Autodesk Inventor part; units mm, degrees
ref_plane "Work Plane1" through (0, 13.97, 1.5) normal (0, 1, 0) x (1, 0, 0)
ref_plane "YZ Plane" through (0, 0, 0) normal (1, 0, 0) x (0, 1, 0)
ref_plane "XZ Plane" through (0, 0, 0) normal (0, 1, 0) x (-1, 0, 0)
sketch "Sketch1" plane through (0, 0, 0) normal (0, 0, 1) x (1, 0, 0)
  line L0 (0, 0) -> (18.04, 0)
  line L1 (18.04, 0) -> (18.04, 27.94) construction
  line L2 (18.04, 27.94) -> (0, 27.94)
  line L3 (0, 27.94) -> (0, 0) construction
  circle A0 centre (9.02, 26.94) radius 0.32
  circle A1 centre (6.48, 26.94) radius 0.32
  circle A2 centre (3.94, 26.94) radius 0.32
  circle A3 centre (11.56, 26.94) radius 0.32
  circle A4 centre (14.1, 26.94) radius 0.32
  circle A5 centre (9.02, 1) radius 0.32
  circle A6 centre (6.48, 1) radius 0.32
  circle A7 centre (3.94, 1) radius 0.32
  circle A8 centre (11.56, 1) radius 0.32
  circle A9 centre (14.1, 1) radius 0.32
  line L4 (-2.665, 23.07) -> (20.705, 23.07) construction
  line L5 (20.705, 23.07) -> (20.705, 4.87) construction
  line L6 (20.705, 4.87) -> (-2.665, 4.87) construction
  line L7 (-2.665, 4.87) -> (-2.665, 23.07) construction
  line L8 (0, 27.94) -> (0, 23.07)
  line L9 (0, 23.07) -> (-2.665, 23.07)
  line L10 (-2.665, 23.07) -> (-2.665, 4.87)
  line L11 (-2.665, 4.87) -> (0, 4.87)
  line L12 (0, 0) -> (0, 4.87)
  line L13 (18.04, 0) -> (18.04, 4.87)
  line L14 (18.04, 4.87) -> (20.705, 4.87)
  line L15 (20.705, 4.87) -> (20.705, 23.07)
  line L16 (20.705, 23.07) -> (18.04, 23.07)
  line L17 (18.04, 23.07) -> (18.04, 27.94)
  point P0 (9.02, 27.94)
  point P1 (9.02, 23.07)
  point P2 (18.04, 13.97)
  point P3 (20.705, 13.97)
  dimension "d0" = 18.04
  dimension "d1" = 27.94
  dimension "d2" = 0.64
  dimension "d3" = 0.64
  dimension "d4" = 2.54
  dimension "d5" = 0.64
  dimension "d6" = 0.64
  dimension "d7" = 0.64
  dimension "d8" = 2.54
  dimension "d9" = 2.54
  dimension "d10" = 2.54
  dimension "d11" = 1
  dimension "d12" = 0.64
  dimension "d13" = 0.64
  dimension "d14" = 2.54
  dimension "d15" = 0.64
  dimension "d16" = 0.64
  dimension "d17" = 0.64
  dimension "d18" = 2.54
  dimension "d19" = 2.54
  dimension "d20" = 2.54
  dimension "d21" = 1
  dimension "d24" = 23.37
  dimension "d25" = 18.2
extrude "Extrusion1" add sketch "Sketch1" along normal blind 1.5
sketch "Sketch2" plane through (0, 0, 1.5) normal (0, 0, 1) x (1, 0, 0)
  line L0 (-2.565, 25.07) -> (20.605, 25.07)
  line L1 (20.605, 25.07) -> (20.605, 2.87)
  line L2 (20.605, 2.87) -> (-2.565, 2.87)
  line L3 (-2.565, 2.87) -> (-2.565, 25.07)
  line L4 (-2.665, 23.07) -> (-2.665, 4.87)
  line L5 (20.705, 4.87) -> (20.705, 23.07)
  line L6 (18.04, 27.94) -> (0, 27.94)
  point P0 (0, 0)
  point P1 (9.02, 25.07)
  point P2 (9.02, 27.94)
  dimension "d27" = 22.2
  dimension "d30" = 0.1
extrude "Extrusion2" add sketch "Sketch2" along normal blind 5.51
sketch "Sketch3" plane through (0, 0, 1.5) normal (0, 0, -1) x (-1, 0, 0)
  line L0 (0, 23.07) -> (2.565, 23.07)
  line L1 (2.565, 23.07) -> (2.565, 25.07)
  line L2 (2.565, 25.07) -> (0, 25.07)
  line L3 (0, 25.07) -> (0, 23.07)
  line L4 (0, 4.87) -> (0, 2.87)
  line L5 (0, 2.87) -> (2.565, 2.87)
  line L6 (2.565, 2.87) -> (2.565, 4.87)
  line L7 (2.565, 4.87) -> (0, 4.87)
  line L8 (-20.605, 23.07) -> (-18.04, 23.07)
  line L9 (-18.04, 23.07) -> (-18.04, 25.07)
  line L10 (-18.04, 25.07) -> (-20.605, 25.07)
  line L11 (-20.605, 25.07) -> (-20.605, 23.07)
  line L12 (-18.04, 2.87) -> (-18.04, 4.87)
  line L13 (-18.04, 4.87) -> (-20.605, 4.87)
  line L14 (-20.605, 4.87) -> (-20.605, 2.87)
  line L15 (-20.605, 2.87) -> (-18.04, 2.87)
  point P0 (0, 0)
extrude "Extrusion3" add sketch "Sketch3" along normal blind 3
sketch "Sketch4" plane through (0, 0, 7.01) normal (0, 0, 1) x (1, 0, 0)
  circle A0 centre (9.02, 13.97) radius 4.5
  line L0 (20.605, 25.07) -> (-2.565, 25.07) construction
  line L1 (-2.565, 25.07) -> (-2.565, 2.87) construction
  line L2 (-2.565, 2.87) -> (20.605, 2.87) construction
  line L3 (20.605, 2.87) -> (20.605, 25.07) construction
  point P0 (0, 0)
  point P1 (9.02, 25.07)
  point P2 (20.605, 13.97)
  dimension "d33" = 9
extrude "Extrusion4" add sketch "Sketch4" along normal blind 6.35
sketch "Sketch5" plane through (9.02, 13.97, 13.36) normal (0, 0, 1) x (1, 0, 0)
  circle A0 centre (0, 0) radius 3.16
  circle A1 centre (0, 0) radius 4.5 construction
  point P0 (-9.02, -13.97)
  dimension "d36" = 6.32
extrude "Extrusion5" add sketch "Sketch5" along normal blind 12.7
sketch "Sketch6" plane through (9.02, 13.97, 26.06) normal (0, 0, 1) x (1, 0, 0)
  line L0 (-3.16, 0.595) -> (3.16, 0.595)
  line L1 (3.16, 0.595) -> (3.16, -0.595)
  line L2 (3.16, -0.595) -> (-3.16, -0.595)
  line L3 (-3.16, -0.595) -> (-3.16, 0.595)
  circle A0 centre (0, 0) radius 3.16 construction
  point P0 (-9.02, -13.97)
  point P1 (3.16, 0)
  point P2 (0, 0.595)
  dimension "d39" = 1.19
extrude "Extrusion6" cut sketch "Sketch6" against normal blind 1.6
thread "Thread1"
fillet "Fillet1" radius 1 1 edges at (4.52, 13.97, 13.36)
fillet "Fillet2" radius 1 4 edges at (20.605, 2.87, 2.755) (-2.565, 2.87, 2.755) (-2.565, 25.07, 2.755) (20.605, 25.07, 2.755)
fillet "Fillet3" radius 1 8 edges at (-2.2721, 24.7771, 7.01) (-2.565, 13.97, 7.01) (-2.2721, 3.1629, 7.01) (9.02, 2.87, 7.01) (20.3121, 3.1629, 7.01) (20.605, 13.97, 7.01) (20.3121, 24.7771, 7.01) (9.02, 25.07, 7.01)
ref_plane "Work Plane1" through (0, 13.97, 1.5) normal (0, 1, 0) x (1, 0, 0)
sketch "Sketch8" plane through (0, 13.97, 1.5) normal (0, 1, 0) x (1, 0, 0)
  line L0 (19.605, -1.51) -> (21.605, -1.51)
  line L1 (19.605, 3) -> (19.605, -4.51) construction
  line L2 (19.605, -1.51) -> (19.605, -5.51)
  line L3 (0, 1.5) -> (18.04, 1.5) construction
  line L4 (9.02, 1.5) -> (9.02, -5.51) construction
  line L5 (19.605, -5.51) -> (-1.565, -5.51) construction
  line L6 (21.605, -1.51) -> (19.605, -5.51)
  line L7 (-1.565, -1.51) -> (-3.565, -1.51)
  line L8 (-1.565, -1.51) -> (-1.565, -5.51)
  line L9 (-3.565, -1.51) -> (-1.565, -5.51)
  dimension "d47" = 2
  dimension "d48" = 4
extrude "Extrusion7" add sketch "Sketch8" along normal mid plane 2.79
sketch "Sketch9" plane through (0, 13.97, 1.5) normal (0, 1, 0) x (1, 0, 0)
  line L0 (-1.565, -5.51) -> (19.605, -5.51)
  line L1 (19.605, -5.51) -> (18.415, -5.51)
  line L2 (18.415, -5.51) -> (18.415, -7.03)
  line L3 (18.415, -7.03) -> (19.605, -7.03)
  line L4 (19.605, -7.03) -> (19.605, -5.51)
  point P0 (0, 1.5)
  dimension "d51" = 1.52
  dimension "d52" = 1.19
extrude "Extrusion8" add sketch "Sketch9" along normal mid plane 2.79
sketch "Sketch10" plane through (0, 0, 7.01) normal (0, 0, 1) x (1, 0, 0)
  circle A0 centre (9.02, 13.97) radius 4.5
  circle A1 centre (9.02, 13.97) radius 7.35
  point P0 (0, 0)
  dimension "d55" = 14.7
extrude "Extrusion9" add sketch "Sketch10" along normal blind 0.25 contours A0 | A1
sketch "Sketch11" plane through (0, 0, 1.5) normal (0, 0, 1) x (1, 0, 0)
  circle A0 centre (9.02, 1) radius 0.32
  circle A1 centre (6.48, 1) radius 0.32
  circle A2 centre (3.94, 1) radius 0.32
  circle A3 centre (11.56, 1) radius 0.32
  circle A4 centre (14.1, 1) radius 0.32
  line L0 (18.04, 2.87) -> (0, 2.87)
  line L1 (0, 2.87) -> (0, 0) construction
  line L2 (0, 0) -> (18.04, 0) construction
  line L3 (18.04, 0) -> (18.04, 2.87) construction
  circle A5 centre (9.02, 26.94) radius 0.32
  circle A6 centre (6.48, 26.94) radius 0.32
  circle A7 centre (3.94, 26.94) radius 0.32
  circle A8 centre (11.56, 26.94) radius 0.32
  circle A9 centre (14.1, 26.94) radius 0.32
  line L4 (0, 25.07) -> (18.04, 25.07) construction
  line L5 (18.04, 25.07) -> (18.04, 27.94) construction
  line L6 (18.04, 27.94) -> (0, 27.94) construction
  line L7 (0, 27.94) -> (0, 25.07) construction
extrude "Extrusion10" add sketch "Sketch11" along normal blind 1 and the other way blind 6.5
equation "\"d2\" = d5"
equation "\"d3\" = d5"
equation "\"d6\" = d5"
equation "\"d7\" = d5"
equation "\"d12\" = d5"
equation "\"d13\" = d5"
equation "\"d15\" = d5"
equation "\"d16\" = d5"
equation "\"d17\" = d5"
equation "\"d21\" = d11"
properties part number "Bourns ACE 128" material "ABS Plastic"
Build history of the part. All positions in model axes, mm. A direction names the side the tool comes from. Round coordinates to 2 decimals unless told otherwise and drop trailing zeros. Order: outer loops, then holes, each group sorted by start corner. A loop starts at its lowest first (then second) coordinate and runs counter-clockwise, first axis right, second up. Notation, with made-up numbers: (-39.75, 55.25) - (-28.75, 55.25) arc R28 ccw to (-28.75, 80.25) - close; hole circle Ø2 at (21, 78). An arc over 180 degrees is marked (long way). Use a Markdown table: item, result.
1) Pull direction X, two halves, no side cores. Call faces 1 (the face through (0, 4, -1)), 2 (the face through (0, 1, 1)), 3 (the face through (18.04, 26, 1)), 4 (the face through (9, 12, 26.06)): pulls with the +X half, pulls with the -X half, needs draft (parallel to the pull), parting line crosses it, or undercut.
Recorded:
| item | result |
|---|---|
| face 1 | undercut |
| face 2 | pulls with the -X half |
| face 3 | pulls with the +X half |
| face 4 | needs draft |
2) Tool access for faces 5 (the face through (9, 9, 7.26)), 6 (the face through (18.04, 4, -1)), 7 (the face through (-1, 23.07, -1)): list every direction of +Z, -Z, +X, -X, +Y, -Y with a clear straight run to the whole face (end or side of a thin tool).
Recorded:
| item | result |
|---|---|
| face 5 | +Z |
| face 6 | -Z, +Y, -Y |
| face 7 | -Z, +X, -X |
3) Saw through at D-D on y = 9. Write the cut outline in (x, z) (3 decimals).
Recorded:
| item | result |
|---|---|
| outline | (-2.665, 0) - (20.705, 0) - (20.705, 1.5) - (20.605, 1.5) - (20.605, 6.01) arc R1 ccw to (19.605, 7.01) - (14.435, 7.01) - (14.435, 7.26) - (3.605, 7.26) - (3.605, 7.01) - (-1.565, 7.01) arc R1 ccw to (-2.565, 6.01) - (-2.565, 1.5) - (-2.665, 1.5) - close |
4) Saw through at A-A on x = 17.5. Write the cut outline in (y, z), and give its area (3 significant figures).
Recorded:
| item | result |
|---|---|
| outline | (0, 0) - (27.94, 0) - (27.94, 1.5) - (25.07, 1.5) - (25.07, 6.01) arc R1 ccw to (24.07, 7.01) - (3.87, 7.01) arc R1 ccw to (2.87, 6.01) - (2.87, 1.5) - (0, 1.5) - close |
| area | 164 mm² |
5) Saw through at C-C on z = 10.5. Write the cut outline in (x, y), and give its area (3 significant figures).
Recorded:
| item | result |
|---|---|
| outline | circle Ø9 at (9.02, 13.97) |
| area | 63.6 mm² |
6) Wall check: L1, parallel to Z at x = 1.75, y = 15.5; L2, parallel to X at y = 21.75, z = 0.5 (3 decimals); L3, parallel to Z at x = 11.25, y = 14.75. Give the ranges that are in metal, low to high.
Recorded:
| item | result |
|---|---|
| L1 | z = 0 to 7.01 |
| L2 | x = -2.665 to 20.705 |
| L3 | z = 0 to 26.06 |
7) Flat gauge pins, fed straight in: pin 1 Ø10 at (y, z) = (11.5, 14.5) entering from +X; pin 2 Ø2 at (x, z) = (14, 7.5) entering from -Y; pin 3 Ø1.2 at (y, z) = (17, 1) entering from -X (3 decimals); pin 4 Ø4 at (x, z) = (10, 2.5) entering from -Y. Where does each tip first touch, or does it go through?
Recorded:
| item | result |
|---|---|
| pin 1 | stops at x = 13.52 |
| pin 2 | stops at y = 3 |
| pin 3 | stops at x = -2.665 |
| pin 4 | stops at y = 0 |
